```python
from build123d import *

# Parameters (mm, degrees)
BOSS_EXTRU_1_DEPTH               = 10
BOSS_EXTRU_2_DEPTH               = 9
CONG_1_R                         = 1.5
R_P_TITION_LIN_AIRE1_COUNT       = 5
R_P_TITION_LIN_AIRE1_PITCH       = 18.5
CONG_1_OF_R_P_TITION_LIN_AIRE1_R = 1.5
ENL_V_MAT_EXTRU_1_DEPTH          = 82.974649169
ENL_V_MAT_EXTRU_1_DEPTH_BACK     = 82.974649169
ESQUISSE4_R                      = 1.5
CONG_2_RADIUS                    = 5
CONG_2_LENGTH                    = 5
CONG_3_RADIUS                    = 5
CONG_3_LENGTH                    = 5
CONG_4_R                         = 10
ESQUISSE5_R                      = 1.5
BOSS_EXTRU_3_DEPTH               = 5
CONG_7_R                         = 2
CONG_8_R                         = 2


with BuildPart() as part:
    # Esquisse1 → Boss.-Extru.1 (new body)
    with BuildSketch(Plane.XY):
        Polygon((-36.5, 10), (36.5, 10), (36.5, -10), (36.5, -15), (41.5, -15), (41.5, 15), (-41.5, 15), (-41.5, -15), (-36.5, -15), (-36.5, -10), align=None)
    extrude(amount=BOSS_EXTRU_1_DEPTH)

    # Esquisse2 → Boss.-Extru.2 (add)
    with BuildSketch(Plane.ZY.offset(41.5)):
        with BuildLine():
            Line((10, 10), (10, 15))
            ThreePointArc((10, 15), (17.110731327, 14.370095429), (24, 12.5))
            ThreePointArc((24, 12.5), (17.110731327, 10.629904571), (10, 10))
        make_face()
    boss_extru_2 = extrude(amount=-BOSS_EXTRU_2_DEPTH)

    # Congé1
    cong_1_edges = [part.edges().sort_by_distance(p)[0] for p in [
        (-37, 12.5, 24),
    ]]
    fillet(cong_1_edges, radius=CONG_1_R)

    # Répétition linéaire1: Boss.-Extru.2 ×5
    with Locations(*[(i * R_P_TITION_LIN_AIRE1_PITCH, 0, 0) for i in range(1, R_P_TITION_LIN_AIRE1_COUNT)]):
        add(boss_extru_2)

    # Congé1 of Répétition linéaire1
    cong_1_of_r_p_tition_lin_aire1_edges = [part.edges().sort_by_distance(p)[0] for p in [
        (-18.5, 12.5, 24),
        (0, 12.5, 24),
        (18.5, 12.5, 24),
        (37, 12.5, 24),
    ]]
    fillet(cong_1_of_r_p_tition_lin_aire1_edges, radius=CONG_1_OF_R_P_TITION_LIN_AIRE1_R)

    # Esquisse4 → Enlèv. mat.-Extru.1 (cut, two sides: drawn at the far end of the back side and taken through both)
    with BuildSketch(Plane(origin=(-36.5, 0, 0), x_dir=(0, 0, -1), z_dir=(1, 0, 0)).offset(-ENL_V_MAT_EXTRU_1_DEPTH_BACK)):
        with Locations((-5, -8)):
            Circle(ESQUISSE4_R)
    extrude(amount=ENL_V_MAT_EXTRU_1_DEPTH + ENL_V_MAT_EXTRU_1_DEPTH_BACK, mode=Mode.SUBTRACT)

    # Congé2: full round fillet: the end face becomes a half cylinder, R = half its width
    cong_2_face = Plane((-39, -15, 5), x_dir=(1, 0, 0), z_dir=(0, -1, 0))  # on the end face: x along it, z out of the body
    cong_2_slab = cong_2_face.offset(-CONG_2_RADIUS / 2) * Box(CONG_2_LENGTH, 2 * CONG_2_RADIUS, CONG_2_RADIUS, mode=Mode.PRIVATE)  # the body's end, R deep
    cong_2_round = Plane((-39, -10, 5), x_dir=(0, -1, 0), z_dir=(1, 0, 0)) * Cylinder(CONG_2_RADIUS, CONG_2_LENGTH, mode=Mode.PRIVATE)  # its axis R under the face
    add(cong_2_slab - cong_2_round, mode=Mode.SUBTRACT)

    # Congé3: full round fillet: the end face becomes a half cylinder, R = half its width
    cong_3_face = Plane((39, -15, 5), x_dir=(1, 0, 0), z_dir=(0, -1, 0))  # on the end face: x along it, z out of the body
    cong_3_slab = cong_3_face.offset(-CONG_3_RADIUS / 2) * Box(CONG_3_LENGTH, 2 * CONG_3_RADIUS, CONG_3_RADIUS, mode=Mode.PRIVATE)  # the body's end, R deep
    cong_3_round = Plane((39, -10, 5), x_dir=(0, -1, 0), z_dir=(1, 0, 0)) * Cylinder(CONG_3_RADIUS, CONG_3_LENGTH, mode=Mode.PRIVATE)  # its axis R under the face
    add(cong_3_slab - cong_3_round, mode=Mode.SUBTRACT)

    # Congé4
    # the kernel refuses this fillet: 10 mm, written as the material it takes off along each edge
    with BuildSketch(Plane(origin=(66.5, 15, 0), x_dir=(0, -1, 0), z_dir=(-1, 0, 0))) as cong_4_piece_1:
        with BuildLine():
            CenterArc((CONG_4_R, CONG_4_R), CONG_4_R, 180, 90)
            Line((0, CONG_4_R), (0, 0))
            Line((0, 0), (CONG_4_R, 0))
        make_face()
    extrude(amount=133, mode=Mode.SUBTRACT)

    # Esquisse5 → Boss.-Extru.3 (add, through all)
    with BuildSketch(Plane(origin=(-36.5, 0, 0), x_dir=(0, 0, -1), z_dir=(1, 0, 0))):
        with BuildLine():
            Line((-14.800353701, -8.485147863), (-11.894696869, -9.209609478))
            ThreePointArc((-11.894696869, -9.209609478), (-11.865496963, -9.365632254), (-11.832766827, -9.520952824))
            Line((-11.832766827, -9.520952824), (-14.240004245, -11.302214812))
            ThreePointArc((-14.240004245, -11.302214812), (-14.404532618, -11.895484958), (-13.868688146, -12.198651174))
            Line((-13.868688146, -12.198651174), (-10.906971813, -11.756019702))
            ThreePointArc((-10.906971813, -11.756019702), (-10.820287286, -11.888991631), (-10.730609975, -12.019963846))
            Line((-10.730609975, -12.019963846), (-12.272947904, -14.586845216))
            ThreePointArc((-12.272947904, -14.586845216), (-12.197917644, -15.197917644), (-11.586845216, -15.272947904))
            Line((-11.586845216, -15.272947904), (-9.019963846, -13.730609975))
            ThreePointArc((-9.019963846, -13.730609975), (-8.888991631, -13.820287286), (-8.756019702, -13.906971813))
            Line((-8.756019702, -13.906971813), (-9.198651174, -16.868688146))
            ThreePointArc((-9.198651174, -16.868688146), (-8.895484958, -17.404532618), (-8.302214812, -17.240004245))
            Line((-8.302214812, -17.240004245), (-6.520952824, -14.832766827))
            ThreePointArc((-6.520952824, -14.832766827), (-6.365632254, -14.865496963), (-6.209609478, -14.894696869))
            Line((-6.209609478, -14.894696869), (-5.485147863, -17.800353701))
            ThreePointArc((-5.485147863, -17.800353701), (-5, -18.179392753), (-4.514852137, -17.800353701))
            Line((-4.514852137, -17.800353701), (-3.790390522, -14.894696869))
            ThreePointArc((-3.790390522, -14.894696869), (-3.634367746, -14.865496963), (-3.479047176, -14.832766827))
            Line((-3.479047176, -14.832766827), (-1.697785188, -17.240004245))
            ThreePointArc((-1.697785188, -17.240004245), (-1.104515042, -17.404532618), (-0.801348826, -16.868688146))
            Line((-0.801348826, -16.868688146), (-1.243980298, -13.906971813))
            ThreePointArc((-1.243980298, -13.906971813), (-1.111008369, -13.820287286), (-0.980036154, -13.730609975))
            Line((-0.980036154, -13.730609975), (1.586845216, -15.272947904))
            ThreePointArc((1.586845216, -15.272947904), (2.197917644, -15.197917644), (2.272947904, -14.586845216))
            Line((2.272947904, -14.586845216), (0.730609975, -12.019963846))
            ThreePointArc((0.730609975, -12.019963846), (0.820287286, -11.888991631), (0.906971813, -11.756019702))
            Line((0.906971813, -11.756019702), (3.868688146, -12.198651174))
            ThreePointArc((3.868688146, -12.198651174), (4.404532618, -11.895484958), (4.240004245, -11.302214812))
            Line((4.240004245, -11.302214812), (1.832766827, -9.520952824))
            ThreePointArc((1.832766827, -9.520952824), (1.865496963, -9.365632254), (1.894696869, -9.209609478))
            Line((1.894696869, -9.209609478), (4.800353701, -8.485147863))
            ThreePointArc((4.800353701, -8.485147863), (5.179392753, -8), (4.800353701, -7.514852137))
            Line((4.800353701, -7.514852137), (1.894696869, -6.790390522))
            ThreePointArc((1.894696869, -6.790390522), (1.865496963, -6.634367746), (1.832766827, -6.479047176))
            Line((1.832766827, -6.479047176), (4.240004245, -4.697785188))
            ThreePointArc((4.240004245, -4.697785188), (4.404532618, -4.104515042), (3.868688146, -3.801348826))
            Line((3.868688146, -3.801348826), (0.906971813, -4.243980298))
            ThreePointArc((0.906971813, -4.243980298), (0.820287286, -4.111008369), (0.730609975, -3.980036154))
            Line((0.730609975, -3.980036154), (2.272947904, -1.413154784))
            ThreePointArc((2.272947904, -1.413154784), (2.197917644, -0.802082356), (1.586845216, -0.727052096))
            Line((1.586845216, -0.727052096), (-0.980036154, -2.269390025))
            ThreePointArc((-0.980036154, -2.269390025), (-1.111008369, -2.179712714), (-1.243980298, -2.093028187))
            Line((-1.243980298, -2.093028187), (-0.801348826, 0.868688146))
            ThreePointArc((-0.801348826, 0.868688146), (-1.104515042, 1.404532618), (-1.697785188, 1.240004245))
            Line((-1.697785188, 1.240004245), (-3.479047176, -1.167233173))
            ThreePointArc((-3.479047176, -1.167233173), (-3.634367746, -1.134503037), (-3.790390522, -1.105303131))
            Line((-3.790390522, -1.105303131), (-4.514852137, 1.800353701))
            ThreePointArc((-4.514852137, 1.800353701), (-5, 2.179392753), (-5.485147863, 1.800353701))
            Line((-5.485147863, 1.800353701), (-6.209609478, -1.105303131))
            ThreePointArc((-6.209609478, -1.105303131), (-6.365632254, -1.134503037), (-6.520952824, -1.167233173))
            Line((-6.520952824, -1.167233173), (-8.302214812, 1.240004245))
            ThreePointArc((-8.302214812, 1.240004245), (-8.895484958, 1.404532618), (-9.198651174, 0.868688146))
            Line((-9.198651174, 0.868688146), (-8.756019702, -2.093028187))
            ThreePointArc((-8.756019702, -2.093028187), (-8.888991631, -2.179712714), (-9.019963846, -2.269390025))
            Line((-9.019963846, -2.269390025), (-11.586845216, -0.727052096))
            ThreePointArc((-11.586845216, -0.727052096), (-12.197917644, -0.802082356), (-12.272947904, -1.413154784))
            Line((-12.272947904, -1.413154784), (-10.730609975, -3.980036154))
            ThreePointArc((-10.730609975, -3.980036154), (-10.820287286, -4.111008369), (-10.906971813, -4.243980298))
            Line((-10.906971813, -4.243980298), (-13.868688146, -3.801348826))
            ThreePointArc((-13.868688146, -3.801348826), (-14.404532618, -4.104515042), (-14.240004245, -4.697785188))
            Line((-14.240004245, -4.697785188), (-11.832766827, -6.479047176))
            ThreePointArc((-11.832766827, -6.479047176), (-11.865496963, -6.634367746), (-11.894696869, -6.790390522))
            Line((-11.894696869, -6.790390522), (-14.800353701, -7.514852137))
            ThreePointArc((-14.800353701, -7.514852137), (-15.179392753, -8), (-14.800353701, -8.485147863))
        make_face()
        with Locations((-5, -8)):
            Circle(ESQUISSE5_R, mode=Mode.SUBTRACT)
    extrude(amount=-BOSS_EXTRU_3_DEPTH)

    # Congé7
    cong_7_edges = [part.edges().sort_by_distance(p)[0] for p in [
        (0, 10, 1.339745962),
    ]]
    fillet(cong_7_edges, radius=CONG_7_R)

    # Congé8
    cong_8_edges = [part.edges().sort_by_distance(p)[0] for p in [
        (-27.75, 15, 10),
        (-9.25, 15, 10),
        (9.25, 15, 10),
        (27.75, 15, 10),
    ]]
    fillet(cong_8_edges, radius=CONG_8_R)


solid = part.part
```
Check sheet for the modelled part. Datum: model origin and axes. Units: mm. A direction names the side the tool comes from. Round coordinates to 2 decimals unless told otherwise and drop trailing zeros. Loops run counter-clockwise (first coordinate to the right, second up) from the corner with the lowest first, then second, coordinate; pieces in that order, holes last. Notation, with made-up numbers: (76, 24) -> (130, 24) arc R19 cw to (130, 31) -> close; hole circle Ø9 at (-26, 49). An arc over 180 degrees is marked (long way). Answer in a Markdown table with one row per item.
Q1. Sectioned sample at B-B on x = 26.5. Enter the section's corners in (y, z), then the cut area to 3 significant figures.
Data:
| item | result |
|---|---|
| outline | (10, 6.13) arc R2 ccw to (13.75, 5.16) arc R10 ccw to (14.68, 7.5) arc R2 ccw to (12.75, 10) -> (10, 10) -> close |
| area | 23.5 mm^2 |
Q2. Sectioned sample at A-A on y = 7.5. Enter the section's corners in (x, z).
Data:
| item | result |
|---|---|
| outline | (-41.5, 0.32) -> (-36.5, 0.32) -> (-36.5, 10) -> (-41.5, 10) -> close; (36.5, 0.32) -> (41.5, 0.32) -> (41.5, 10) -> (36.5, 10) -> close |
Q3. Release check for a two-part mould opening along Z. For faces 1 (the face through (-38.965, -11.974, -2.367)), 2 (the face through (-38.97, -5.6, -3.02)), 3 (the face through (-41.5, -1, 5)), 4 (the face through (-38.97, -5.58, 13.05)) record: released by +Z, released by -Z, zero draft, split by the parting line, or undercut.
Data:
| item | result |
|---|---|
| face 1 | undercut |
| face 2 | released by -Z |
| face 3 | zero draft |
| face 4 | released by +Z |
Q4. Thickness scan on L1, parallel to X at y = 13, z = 15.5; L2, parallel to Z at x = 39, y = -8; L3, parallel to X at y = 0.5, z = 1.5. Record the ranges inside material, lowest first.
Data:
| item | result |
|---|---|
| L1 | x = -41.5 to -32.5, -23 to -14, -4.5 to 4.5, 14 to 23, 32.5 to 41.5 |
| L2 | z = 0 to 3.5, 6.5 to 10 |
| L3 | x = -41.5 to -36.5, 36.5 to 41.5 |
Q5. Set-up check for faces 5 (the face through (-38.97, -7.16, -3.37)), 6 (the face through (-38.97, -8.84, 13.37)), 7 (the face through (28, 11, 10)), 8 (the face through (-38.97, -16.02, 2.6)), 9 (the face through (39, -2, 0)): record each of +Z, -Z, +X, -X, +Y, -Y from which the full face is reachable in a straight line by a thin tool's end or side.
Data:
| item | result |
|---|---|
| face 5 | -Z, +X, -X |
| face 6 | +Z, +X, -X |
| face 7 | +Z, +Y, -Y |
| face 8 | +X, -X, -Y |
| face 9 | -Z, +X, +Y, -Y |
Q6. Go/stop test with flat-tipped pins: P1, Ø8, axis at x = -13.5, z = 13, coming from the -Y side; P2, Ø2, axis at x = -10, y = 12, coming from the +Z side; P3, Ø5, axis at x = 29, z = 2.5, coming from the -Y side. Record where each tip stops, or that it passes through.
Data:
| item | result |
|---|---|
| P1 | stops at y = 10 |
| P2 | stops at z = 10 |
| P3 | stops at y = 10.35 |
